Read the model definition and answer for the solid it produces. Units are mm, in the model's axes. A direction names the side the tool comes from. Coordinates: 2 decimals unless noted, no trailing zeros. Write each loop counter-clockwise with the first axis right and the second up, starting at its lowest first coordinate (ties: lowest second). Pieces come first, ordered by that corner, then holes. Notation, with made-up numbers: (4, -18) -> (10, -18) arc R27 ccw to (10, 4) -> close; hole circle Ø8 at (11, -9.5). An arc over 180 degrees is marked (long way). Use CSV: the item, a comma, the result in double quotes.
from build123d import *

# Parameters (mm, degrees)
F1_DEPTH = 12.7
F2_W     = 4.7
F2_H     = 35
F3_DEPTH = 1
F4_R     = 2


with BuildPart() as f1:
    # F0 (on Right) → F1 (new body, symmetric)
    with BuildSketch(Plane.YZ):
        Polygon((6.7, 0), (0, 0), (0, -42), (1, -42), (1, -1), (5.7, -1), (5.7, -3.5), (6.7, -3.5), align=None)
    extrude(amount=F1_DEPTH, both=True)

    # F2 (on face) → F3 (cut, through all)
    with BuildSketch(Plane.XZ):
        Polygon((3.1, 0), (-3.1, 0), (-3.1, -33), (-4, -38), (4, -38), (3.1, -33), align=None)
        with Locations((-10.35, -24.5)):
            Rectangle(F2_W, F2_H)
        with Locations((10.35, -24.5)):
            Rectangle(F2_W, F2_H)
    extrude(amount=-F3_DEPTH, mode=Mode.SUBTRACT)

    # F4
    f4_edges = [f1.edges().sort_by_distance(p)[0] for p in [
        (8, 0.5, -42),
        (-8, 0.5, -42),
        (-8, 0.5, -7),
        (-12.7, 0.5, -7),
        (8, 0.5, -7),
        (12.7, 0.5, -7),
    ]]
    fillet(f4_edges, radius=F4_R)


solid = f1.part
1. A cutting plane is placed at D-D (y = 6.25). Give the vertices of the cut face in (x, z), and give its area (3 significant figures).
Solutions:
outline,"(-12.7, -3.5) -> (12.7, -3.5) -> (12.7, 0) -> (-12.7, 0) -> close"
area,"88.9 mm^2"
2. A cutting plane is placed at A-A (z = -36.5). Give the vertices of the cut face in (x, y), and give its area (3 significant figures).
Solutions:
outline,"(-8, 0) -> (-3.73, 0) -> (-3.73, 1) -> (-8, 1) -> close; (3.73, 0) -> (8, 0) -> (8, 1) -> (3.73, 1) -> close"
area,"8.54 mm^2"
3. For a pull along Z with two mould halves and no side action, classify faces 5 (the flat face through (3.556, 0.493, -35.535)), 6 (the flat face through (-8, 0.5, -24.7)), 7 (the cylindrical face through (-12.13, 0.51, -6.4)) as pulls with the +Z half, pulls with the -Z half, needs draft (parallel to the pull), parting line crosses it, or undercut.
Solutions:
face 5,"undercut"
face 6,"needs draft"
face 7,"pulls with the -Z half"
4. A cutting plane is placed at C-C (z = -19). Give the vertices of the cut face in (x, y), and give its area (3 significant figures).
Solutions:
outline,"(-8, 0) -> (-3.1, 0) -> (-3.1, 1) -> (-8, 1) -> close; (3.1, 0) -> (8, 0) -> (8, 1) -> (3.1, 1) -> close"
area,"9.80 mm^2"
5. A tool of negligible diameter and unlimited length cuts with its end or side. For faces 1 (the flat face through (-4, 1, -22)), 2 (the flat face through (8, 0.5, -24.7)), 3 (the flat face through (0, 6, -3.5)), 4 (the flat face through (-0.1, 0.5, -38)), from which of +Z, -Z, +X, -X, +Y, -Y can it reach the whole face along a straight path? Write none if from no direction.
Solutions:
face 1,"-Z, +X, -X"
face 2,"-Z, +X, +Y, -Y"
face 3,"-Z, +X, -X, +Y"
face 4,"+Y, -Y"
6. Find the intervals of material crossed by line 1 along Z through (x, y) = (2.75, 1.75); line 2 along Y through (x, z) = (-5.25, -6); line 3 along Z through (x, y) = (7.25, 5.75), in increasing order.
Solutions:
line 1,"z = -1 to 0"
line 2,"y = 0 to 1"
line 3,"z = -3.5 to 0"
7. Each of these flat-tipped pins is pushed along its axis until it touches: pin 1 Ø0.5 at (y, z) = (0.5, -12) entering from +X; pin 2 Ø0.5 at (x, z) = (-0.5, -0.5) entering from -Y; pin 3 Ø4 at (x, y) = (-4.5, 4.5) entering from -Z. Where does it stop, or does it pass through?
Solutions:
pin 1,"stops at x = 8"
pin 2,"stops at y = 1"
pin 3,"stops at z = -3.5"
8. A cutting plane is placed at B-B (x = -5.5). Give the vertices of the cut face in (y, z), and give its area (3 significant figures).
Solutions:
outline,"(0, -42) -> (1, -42) -> (1, -1) -> (5.7, -1) -> (5.7, -3.5) -> (6.7, -3.5) -> (6.7, 0) -> (0, 0) -> close"
area,"50.2 mm^2"
